```python
from build123d import *

# Parameters (mm, degrees)
BOSS_EXTRUDE1_DEPTH = 15
SKETCH2_R           = 10
BOSS_EXTRUDE2_DEPTH = 134
SKETCH4_R           = 7.25
CUT_EXTRUDE1_DEPTH  = 57
SKETCH5_R           = 5
CUT_EXTRUDE2_DEPTH  = 93
SKETCH7_R           = 6.5
CUT_EXTRUDE3_DEPTH  = 6.6
SKETCH8_R           = 3.3
CUT_EXTRUDE4_DEPTH  = 9.4
SKETCH9_R           = 3
CUT_EXTRUDE5_DEPTH  = 16
FILLET1_R           = 1
FILLET2_R           = 0.5
SKETCH10_R          = 2
CUT_EXTRUDE11_DEPTH = 48


with BuildPart() as part:
    # Sketch1 → Boss-Extrude1 (new body)
    with BuildSketch(Plane(origin=(0, 0, 0), x_dir=(1, 0, 0), z_dir=(0, 1, 0))):
        with BuildLine():
            Line((17, -24.718414189), (17, 24.718414189))
            ThreePointArc((17, 24.718414189), (-30, 0), (17, -24.718414189))
        make_face()
    extrude(amount=BOSS_EXTRUDE1_DEPTH)

    # Sketch2 → Boss-Extrude2 (add)
    with BuildSketch(Plane(origin=(0, 15, 0), x_dir=(1, 0, 0), z_dir=(0, 1, 0))):
        Circle(SKETCH2_R)
    extrude(amount=BOSS_EXTRUDE2_DEPTH)

    # Sketch4 → Cut-Extrude1 (cut)
    with BuildSketch(Plane.XZ):
        Circle(SKETCH4_R)
    extrude(amount=-CUT_EXTRUDE1_DEPTH, mode=Mode.SUBTRACT)

    # Sketch5 → Cut-Extrude2 (cut, through all)
    with BuildSketch(Plane.XZ.offset(-57)):
        Circle(SKETCH5_R)
    extrude(amount=-CUT_EXTRUDE2_DEPTH, mode=Mode.SUBTRACT)

    # Sketch7 → Cut-Extrude3 (cut)
    with BuildSketch(Plane(origin=(0, 15, 0), x_dir=(1, 0, 0), z_dir=(0, 1, 0))):
        with Locations((0, -20)):
            Circle(SKETCH7_R)
        with Locations((-20, 0)):
            Circle(SKETCH7_R)
        with Locations((0, 20)):
            Circle(SKETCH7_R)
    extrude(amount=-CUT_EXTRUDE3_DEPTH, mode=Mode.SUBTRACT)

    # Sketch8 → Cut-Extrude4 (cut, through all)
    with BuildSketch(Plane(origin=(0, 8.4, 0), x_dir=(1, 0, 0), z_dir=(0, 1, 0))):
        with Locations((0, -20)):
            Circle(SKETCH8_R)
        with Locations((-20, 0)):
            Circle(SKETCH8_R)
        with Locations((0, 20)):
            Circle(SKETCH8_R)
    extrude(amount=-CUT_EXTRUDE4_DEPTH, mode=Mode.SUBTRACT)

    # Sketch9 → Cut-Extrude5 (cut, through all)
    with BuildSketch(Plane(origin=(0, 15, 0), x_dir=(1, 0, 0), z_dir=(0, 1, 0))):
        with Locations((-10.606601718, -10.606601718)):
            Circle(SKETCH9_R)
        with Locations((10.606601718, 10.606601718)):
            Circle(SKETCH9_R)
    extrude(amount=-CUT_EXTRUDE5_DEPTH, mode=Mode.SUBTRACT)

    # Fillet1
    fillet1_edges = [part.edges().sort_by_distance(p)[0] for p in [
        (17, 7.5, -24.718414189),
        (17, 7.5, 24.718414189),
    ]]
    fillet(fillet1_edges, radius=FILLET1_R)

    # Fillet2
    fillet2_edges = [part.edges().sort_by_distance(p)[0] for p in [
        (-10, 149, 0),
    ]]
    fillet(fillet2_edges, radius=FILLET2_R)

    # Sketch10 → Cut-Extrude11 (cut, through all)
    with BuildSketch(Plane(origin=(17, 0, 0), x_dir=(0, 0, -1), z_dir=(1, 0, 0))):
        with Locations((-5, 82)):
            Circle(SKETCH10_R)
    extrude(amount=-CUT_EXTRUDE11_DEPTH, mode=Mode.SUBTRACT)


solid = part.part
```
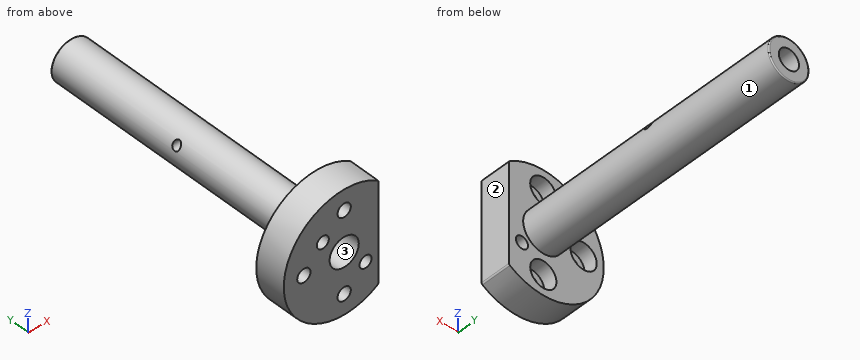
Work out the finished part from the listing and answer in its coordinate system (mm). Face numbers are marked on the shaded views. Give positions to 0.01 mm unless a question says otherwise; leave off trailing zeros. Loops run counter-clockwise (first coordinate to the right, second up) from the corner with the lowest first, then second, coordinate; pieces in that order, holes last. Notation, with made-up numbers: M -11.75,54 L -4.75,54 A22 ccw -4.75,80 Z; hole C 86.25,-27.75 d10. An arc over 180 degrees is marked long. One line per item, written item: value. Start each with the question number.
1. Determine the mould class of the marked faces 1, 2 and 3 for opening direction X: released by +X, released by -X, zero draft, split by the parting line, or undercut.
2. Find section C-C (y = 82). Give the vertices of the cut face in (x, z).
3. Each of these flat-tipped pins is pushed along its axis until it touches: P1, Ø4, axis at x = -20, z = 0, coming from the +Y side (3 decimals); P2, Ø10.5, axis at x = -21, z = -3, coming from the +Y side; P3, Ø5, axis at x = -8.5, y = 128, coming from the -Z side; P4, Ø6, axis at x = 3, y = 40.5, coming from the -Z side. Where does it stop, or does it pass through?
4. Find section B-B (y = 38). Give the vertices of the cut face in (x, z).
5. Find section A-A (z = 20). Give the vertices of the cut face in (x, y), and give its area (3 significant figures).
6. Find section D-D (y = 133.5). Give the vertices of the cut face in (x, z).
7. Find the intervals of material crossed by probe 1 along Z at (x, y) = (0, 5); probe 2 along Z at (x, y) = (0, 82); probe 3 along Z at (x, y) = (0, 33), in increasing order.
Reported:
1. face 1: split by the parting line
1. face 2: released by +X
1. face 3: undercut
2. outline: M -9.54,3 A10 ccw long 9.54,3 L 4,3 A5 cw long -4,3 Z; M -7.14,7 L 7.14,7 A10 ccw Z
3. P1: passes through
3. P2: stops at y = 15
3. P3: stops at z = -8
3. P4: stops at z = -10
4. outline: C 0,0 d20; hole C 0,0 d14.5
5. outline: M -22.36,0 L -3.3,0 L -3.3,8.4 L -6.5,8.4 L -6.5,15 L -22.36,15 Z; M 3.3,0 L 17,0 L 17,15 L 6.5,15 L 6.5,8.4 L 3.3,8.4 Z
5. area: 449 mm²
6. outline: C 0,0 d20; hole C 0,0 d10
7. probe 1: z = -30 to -23.3, -16.7 to -7.25, 7.25 to 16.7, 23.3 to 30
7. probe 2: z = -10 to -5, 7 to 10
7. probe 3: z = -10 to -7.25, 7.25 to 10
